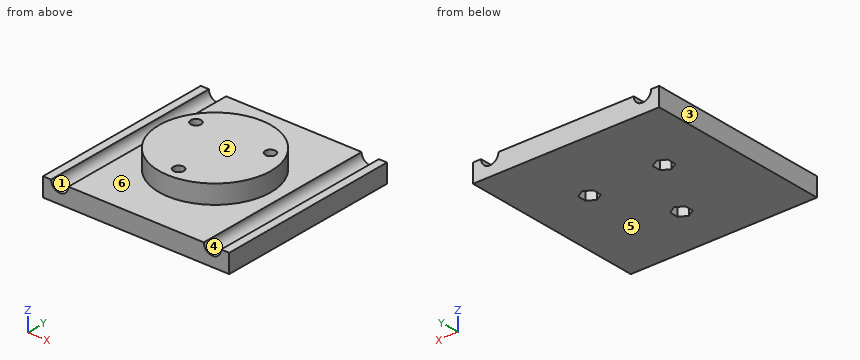
```python
from build123d import *

# Parameters (mm, degrees)
F0_W     = 100
F0_H     = 100
F1_DEPTH = 10
F2_R     = 4.65
F3_DEPTH = 100.001
F4_R     = 30
F5_DEPTH = 10
F7_DEPTH = 20.001
F8_R     = 2.8
F9_DEPTH = 5


with BuildPart() as f1:
    # F0 (on Top) → F1 (new body)
    with BuildSketch(Plane.XY):
        Rectangle(F0_W, F0_H)
    extrude(amount=F1_DEPTH)

    # F2 (on face) → F3 (cut, through all)
    with BuildSketch(Plane.XZ.offset(50)):
        with Locations((-41, 10)):
            Circle(F2_R)
        with Locations((41, 10)):
            Circle(F2_R)
    extrude(amount=-F3_DEPTH, mode=Mode.SUBTRACT)

    # F4 (on face) → F5 (join)
    with BuildSketch(Plane.XY.offset(10)):
        Circle(F4_R)
    extrude(amount=F5_DEPTH)

    # F6 (on face) → F7 (cut, through all)
    with BuildSketch(Plane.XY.offset(20)):
        with BuildLine():
            ThreePointArc((-18.6, 9.122134), (-17.575129, 10.147005), (-17.2, 11.547005))
            Line((-17.2, 11.547005), (-20, 11.547005))
            Line((-20, 11.547005), (-18.6, 9.122134))
        make_face()
        with BuildLine():
            Line((-20, 11.547005), (-17.2, 11.547005))
            ThreePointArc((-17.2, 11.547005), (-22.424871, 12.947005), (-18.6, 9.122134))
            Line((-18.6, 9.122134), (-20, 11.547005))
        make_face()
        with BuildLine():
            Line((18.6, 9.122134), (20, 11.547005))
            Line((20, 11.547005), (17.2, 11.547005))
            ThreePointArc((17.2, 11.547005), (17.575129, 10.147005), (18.6, 9.122134))
        make_face()
        with BuildLine():
            Line((17.2, 11.547005), (20, 11.547005))
            Line((20, 11.547005), (18.6, 9.122134))
            ThreePointArc((18.6, 9.122134), (21.4, 9.122134), (22.8, 11.547005))
            ThreePointArc((22.8, 11.547005), (20, 14.347005), (17.2, 11.547005))
        make_face()
        with BuildLine():
            Line((0, -23.094011), (1.4, -20.66914))
            ThreePointArc((1.4, -20.66914), (0, -20.294011), (-1.4, -20.66914))
            Line((-1.4, -20.66914), (0, -23.094011))
        make_face()
        with BuildLine():
            ThreePointArc((2.8, -23.094011), (2.424871, -21.694011), (1.4, -20.66914))
            Line((1.4, -20.66914), (0, -23.094011))
            Line((0, -23.094011), (-1.4, -20.66914))
            ThreePointArc((-1.4, -20.66914), (-1.4, -25.518882), (2.8, -23.094011))
        make_face()
    extrude(amount=-F7_DEPTH, mode=Mode.SUBTRACT)

    # F8 (on face) → F9 (cut)
    with BuildSketch(Plane(origin=(0, 0, 0), x_dir=(1, 0, 0), z_dir=(0, 0, -1))):
        Polygon((0, 18.359739), (4.1, 20.726875), (4.1, 25.461147), (0, 27.828283), (-4.1, 25.461147), (-4.1, 20.726875), align=None)
        with Locations((0, 23.094011)):
            Circle(F8_R, mode=Mode.SUBTRACT)
        Polygon((-20, -16.281278), (-15.9, -13.914141), (-15.9, -9.179869), (-20, -6.812733), (-24.1, -9.179869), (-24.1, -13.914141), align=None)
        with Locations((-20, -11.547005)):
            Circle(F8_R, mode=Mode.SUBTRACT)
        Polygon((20, -16.281278), (24.1, -13.914141), (24.1, -9.179869), (20, -6.812733), (15.9, -9.179869), (15.9, -13.914141), align=None)
        with Locations((20, -11.547005)):
            Circle(F8_R, mode=Mode.SUBTRACT)
    extrude(amount=-F9_DEPTH, mode=Mode.SUBTRACT)


solid = f1.part
```
For this review, take the finished solid that the model builds, in its own axes (mm). Face numbers are marked on the shaded views. A direction names the side the tool comes from. Round coordinates to 2 decimals unless told otherwise and drop trailing zeros. Order: outer loops, then holes, each group sorted by start corner. A loop starts at its lowest first (then second) coordinate and runs counter-clockwise, first axis right, second up.
Q1. Insertion check: P1, Ø5, axis at x = 48.5, y = 13.5, coming from the +Z side; P2, Ø4, axis at x = 1.5, y = -23, coming from the -Z side. Each pin has a flat end and moves straight along its axis. Give the tip position at first contact, or say it passes through.
Findings below:
P1: stops at z = 10
P2: stops at z = 5
Q2. Mouldability with a two-part tool opening along X and no side actions: class the marked faces 1, 2, 3 and 4 as pulls with the +X half, pulls with the -X half, needs draft (parallel to the pull), parting line crosses it, or undercut.
Findings below:
face 1: undercut
face 2: needs draft
face 3: pulls with the -X half
face 4: undercut
Q3. Wall thickness on line 1 (Y direction, x = 0, z = 13.75); line 2 (X direction, y = 17, z = 7.75); line 3 (Y direction, x = 0, z = 9.25): over which ranges is each line inside the solid? List them lowest first.
Findings below:
line 1: y = -30 to -25.89, -20.29 to 30
line 2: x = -50 to -45.07, -36.93 to 36.93, 45.07 to 50
line 3: y = -50 to -25.89, -20.29 to 50
Q4. We need section C-C, the plane x = -41. Give the boundary of the cut face in (y, z), plus the area to 3 significant figures.
Findings below:
outline: (-50, 0) - (50, 0) - (50, 5.35) - (-50, 5.35) - close
area: 535 mm2
Q5. We need section A-A, the plane z = 3.75. Give the boundary of the cut face in (x, y).
Findings below:
outline: (-50, -50) - (50, -50) - (50, 50) - (-50, 50) - close; hole (-24.1, 9.18) - (-20, 6.81) - (-15.9, 9.18) - (-15.9, 13.91) - (-20, 16.28) - (-24.1, 13.91) - close; hole (-4.1, -25.46) - (0, -27.83) - (4.1, -25.46) - (4.1, -20.73) - (0, -18.36) - (-4.1, -20.73) - close; hole (15.9, 9.18) - (20, 6.81) - (24.1, 9.18) - (24.1, 13.91) - (20, 16.28) - (15.9, 13.91) - close
Q6. Machinability: for the marked faces 5 and 6, which of the approach directions +Z, -Z, +X, -X, +Y, -Y give a long, thin tool a straight path to every point of the face, cutting with its end or side? Answer none if there is none.
Findings below:
face 5: -Z, +X, -X, +Y, -Y
face 6: +Z
Q7. We need section D-D, the plane y = 38. Give the boundary of the cut face in (x, z).
Findings below:
outline: (-50, 0) - (50, 0) - (50, 10) - (45.65, 10) arc R4.65 cw to (36.35, 10) - (-36.35, 10) arc R4.65 cw to (-45.65, 10) - (-50, 10) - close
Q8. We need section B-B, the plane y = 0. Give the boundary of the cut face in (x, z).
Findings below:
outline: (-50, 0) - (50, 0) - (50, 10) - (45.65, 10) arc R4.65 cw to (36.35, 10) - (30, 10) - (30, 20) - (-30, 20) - (-30, 10) - (-36.35, 10) arc R4.65 cw to (-45.65, 10) - (-50, 10) - close
